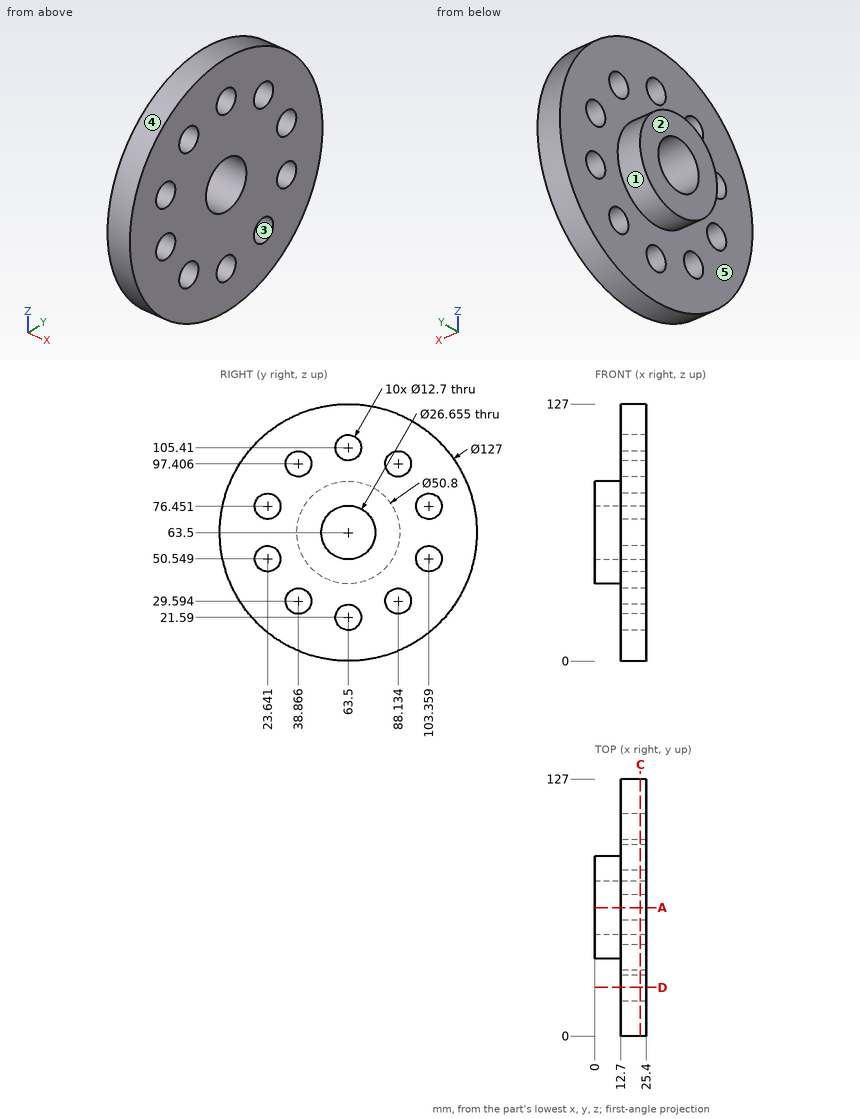
Geometry check sheet. Reference: drawing and pictorial views, mm from the part's lowest x, y, z. A direction names the side the tool comes from. Give positions to 0.01 mm unless a question says otherwise; leave off trailing zeros. Write each loop counter-clockwise with the first axis right and the second up, starting at its lowest first coordinate (ties: lowest second). Pieces come first, ordered by that corner, then holes. Notation, with made-up numbers: M -30.75,-11.5 L -25.75,-11.5 A21 cw -25.75,14.5 Z; hole C 37,68 d1. An arc over 180 degrees is marked long. Put each result on its own line as item: value. Start each with the question number.
1. Section check C-C (x = 22.5). Give the number of separate pieces and of enclosed holes in the cut face, and give its area (3 significant figures).
2. Section check A-A (y = 63.5). Record the cut outline in (x, z), and give its area (3 significant figures).
3. Set-up check for the marked faces 4 and 5: record each of +Z, -Z, +X, -X, +Y, -Y from which the full face is reachable in a straight line by a thin tool's end or side.
4. Scan lines: line 1 along Z through (x, y) = (13, 93) (1 decimal); line 2 along Y through (x, z) = (21.5, 54) (1 decimal); line 3 along Y through (x, z) = (19, 63.5). Record each from-to range of solid material in increasing order. Write a range as [from, to].
5. Section check D-D (y = 24). Record the cut outline in (x, z).
6. Go/stop test with flat-tipped pins: pin 1 Ø4 at (x, y) = (9.5, 74) entering from -Z (1 decimal); pin 2 Ø16.5 at (y, z) = (23.64, 50.55) entering from -X; pin 3 Ø14.5 at (y, z) = (38.87, 97.41) entering from +X; pin 4 Ø6 at (x, y) = (18.5, 69.5) entering from +Z. Record where each tip stops, or that it passes through.
7. Draft check along Y on the marked faces 1, 2 and 3. Enter one of: +Y half, -Y half, draft (parallel to the pull), parting line (faces both ways), or undercut.
Answer list:
1. separate pieces: 1
1. enclosed holes: 11
1. area: 10,800 mm2
2. outline: M 0,38.1 L 12.7,38.1 L 12.7,27.94 L 25.4,27.94 L 25.4,50.17 L 0,50.17 Z; M 0,76.83 L 25.4,76.83 L 25.4,99.06 L 12.7,99.06 L 12.7,88.9 L 0,88.9 Z; M 12.7,0 L 25.4,0 L 25.4,15.24 L 12.7,15.24 Z; M 12.7,111.76 L 25.4,111.76 L 25.4,127 L 12.7,127 Z
2. area: 1,260 mm2
3. face 4: +X, -X
3. face 5: -X
4. line 1: [7.3, 25.5], [33.7, 93.3], [101.5, 119.7]
4. line 2: [0.7, 18.3], [29, 54.2], [72.8, 98], [108.7, 126.3]
4. line 3: [0, 50.17], [76.83, 127]
5. outline: M 12.7,13.78 L 25.4,13.78 L 25.4,44.21 L 12.7,44.21 Z; M 12.7,56.89 L 25.4,56.89 L 25.4,70.11 L 12.7,70.11 Z; M 12.7,82.79 L 25.4,82.79 L 25.4,113.22 L 12.7,113.22 Z
6. pin 1: z = 39.6
6. pin 2: x = 12.7
6. pin 3: x = 25.4
6. pin 4: z = 126.93
7. face 1: parting line
7. face 2: draft
7. face 3: undercut
